Verification items for the finished model (mm, model axes). A direction names the side the tool comes from. Coordinates: 2 decimals unless noted, no trailing zeros. Loops run counter-clockwise (first coordinate to the right, second up) from the corner with the lowest first, then second, coordinate; pieces in that order, holes last. Notation, with made-up numbers: (-17, 58.5) - (22, 58.5) arc R19 cw to (22, 82.5) - close; hole circle Ø4 at (35, 65). An arc over 180 degrees is marked (long way). One line per item, written item: value. Start each with the question number.
(1) Thickness scan on probe 1 along X at (y, z) = (-18.5, 1.5); probe 2 along X at (y, z) = (-6, 2); probe 3 along Y at (x, z) = (47.5, 1.5). Record the ranges inside material, lowest first. Write a range as [from, to].
(2) Section check B-B (x = 33.5). Record the boundary of the cut face in (y, z), plus the area to 3 significant figures.
(3) Section check D-D (z = 1.5). Count the separate pieces of the cut face and the enclosed holes in it, plus the area to 3 significant figures.
(4) Set-up check for faces 5 (the face through (61, -1.707, 1)), 6 (the face through (16.99, 9.74, 1.46)), 7 (the face through (69.238, 16.323, -0.677)), 8 (the face through (24, 9.901, 1)), 9 (the face through (37.1, 12.4, 0)): record each of +Z, -Z, +X, -X, +Y, -Y from which the full face is reachable in a straight line by a thin tool's end or side.
(5) Section check C-C (x = 61.5). Record the boundary of the cut face in (y, z).
(6) Draft check along X on faces 1 (the face through (69.953, 9, 1)), 2 (the face through (25, -1.707, 1)), 3 (the face through (69.24, 9.74, 1.54)), 4 (the face through (61.747, -8.946, 1.351)). Enter one of: +X half, -X half, draft (parallel to the pull), parting line (faces both ways), or undercut.
(7) Gauge pin test, flat ends, axial feed: P1, Ø1, axis at x = 36, y = 18, coming from the +Z side; P2, Ø2, axis at x = 62, z = 1.5, coming from the -Y side; P3, Ø1.5, axis at y = 0, z = 2, coming from the +X side; P4, Ø8, axis at x = 37, y = -7.5, coming from the +Z side. Record the tip position at first contact, or that the pin passes through.
(8) Section check A-A (x = 25). Record the boundary of the cut face in (y, z), plus the area to 3 significant figures.
```python
from build123d import *

# Parameters (mm, degrees)
SKETCH_1_R          = 15
SKETCH_1_R_2        = 1.4
EXTRUDE_1_DEPTH     = 2.74
SKETCH_3_W          = 2.74
SKETCH_3_H          = 6
EXTRUDE_3_DEPTH     = 3.5
SKETCH_11_W         = 2.74
SKETCH_11_H         = 6
EXTRUDE_8_DEPTH     = 3.5
FILLET_17_R         = 2
FILLET_19_R         = 2
CUT_EXTRUDE_1_DEPTH = 1.45
CUT_EXTRUDE_START   = -1.45
CUT_EXTRUDE_2_DEPTH = 1.45


with BuildPart() as part:
    # 草图1 → 凸台-拉伸1 (new body)
    with BuildSketch(Plane.XY):
        with BuildLine():
            Line((25.602982383, 9.901284161), (25.602982383, 3.901284161))
            Line((25.602982383, 3.901284161), (22.865684115, 3.901284161))
            ThreePointArc((22.865684115, 3.901284161), (43.102982383, -22.706902605), (63.340280651, 3.901284161))
            Line((63.340280651, 3.901284161), (60.602982383, 3.901284161))
            Line((60.602982383, 3.901284161), (60.602982383, 9.901284161))
            ThreePointArc((60.602982383, 9.901284161), (43.102982383, 19.293097395), (25.602982383, 9.901284161))
        make_face()
        with Locations((43.102982383, -1.706902605)):
            Circle(SKETCH_1_R, mode=Mode.SUBTRACT)
        with Locations((38.37953481, 15.921243725)):
            Circle(SKETCH_1_R_2, mode=Mode.SUBTRACT)
        with Locations((47.826429956, -19.335048935)):
            Circle(SKETCH_1_R_2, mode=Mode.SUBTRACT)
        with BuildLine():
            Line((26.602982383, -1.706902605), (23.102982383, -1.706902605))
            ThreePointArc((23.102982383, -1.706902605), (28.96084676, -15.849038229), (43.102982383, -21.706902605))
            Line((43.102982383, -21.706902605), (43.102982383, -18.206902605))
            ThreePointArc((43.102982383, -18.206902605), (31.435720494, -13.374164495), (26.602982383, -1.706902605))
        make_face(mode=Mode.SUBTRACT)
        with BuildLine():
            Line((43.102982383, 14.793097395), (43.102982383, 18.12026115))
            ThreePointArc((43.102982383, 18.12026115), (52.478832846, 15.763353566), (59.625618846, 9.252974534))
            Line((59.625618846, 9.252974534), (56.852982383, 7.413815568))
            ThreePointArc((56.852982383, 7.413815568), (50.905486793, 12.831698598), (43.102982383, 14.793097395))
        make_face(mode=Mode.SUBTRACT)
        with BuildLine():
            Line((55.393395475, -12.715796557), (58.000452797, -15.051016486))
            ThreePointArc((58.000452797, -15.051016486), (61.783847035, -8.850101879), (63.102982383, -1.706902605))
            Line((63.102982383, -1.706902605), (59.602982383, -1.706902605))
            ThreePointArc((59.602982383, -1.706902605), (58.514695721, -7.600042006), (55.393395475, -12.715796557))
        make_face(mode=Mode.SUBTRACT)
    extrude(amount=EXTRUDE_1_DEPTH)

    # 草图3 → 凸台-拉伸3 (add)
    with BuildSketch(Plane.ZY.offset(-25.602982383)):
        with Locations((1.37, 6.901284161)):
            Rectangle(SKETCH_3_W, SKETCH_3_H)
    extrude(amount=EXTRUDE_3_DEPTH)

    # 草图11 → 凸台-拉伸8 (add)
    with BuildSketch(Plane(origin=(60.602982383, 0, 0), x_dir=(0, 0, -1), z_dir=(1, 0, 0))):
        with Locations((-1.37, 6.901284161)):
            Rectangle(SKETCH_11_W, SKETCH_11_H)
    extrude(amount=EXTRUDE_8_DEPTH)

    # 圆角17
    # the kernel refuses this fillet: 2 mm, written as the material it adds along each edge
    with BuildSketch(Plane(origin=(63.340280651, 3.901284161, 0), x_dir=(0.228936975336042, -0.9734412469810308, 0), z_dir=(0, 0, 1))) as fillet_17_piece_1:
        with BuildLine():
            CenterArc((1.731032211, 1.998451636), FILLET_17_R, 218.902952144, 48.842355981)
            Line((0.174610628, 0.742445325), (0.143482196, 0.717325199))
            ThreePointArc((0.143482196, 0.717325199), (0.048367664, 0.380380141), (-0.03893765, 0.009157479))
            Line((-0.03893765, 0.009157479), (0.001573666, -0.039969033))
            ThreePointArc((0.001573666, -0.039969033), (0.826174465, -0.023742177), (1.650775263, -0.039969033))
            Line((1.650775263, -0.039969033), (1.652348929, 0))
        make_face()
    extrude(amount=2.74)

    # 圆角19
    # the kernel refuses this fillet: 2 mm, written as the material it adds along each edge
    with BuildSketch(Plane(origin=(22.865684115, 3.901284161, 0), x_dir=(-0.22893697533604487, -0.9734412469810302, 0), z_dir=(0, 0, 1))) as fillet_19_piece_1:
        with BuildLine():
            CenterArc((1.731032211, -1.998451636), FILLET_19_R, 92.254691875, 48.842355981)
            Line((0.174610628, -0.742445325), (0.143482196, -0.717325199))
            ThreePointArc((0.143482196, -0.717325199), (0.048367664, -0.380380141), (-0.03893765, -0.009157479))
            Line((-0.03893765, -0.009157479), (0.001573666, 0.039969033))
            ThreePointArc((0.001573666, 0.039969033), (0.826174465, 0.023742177), (1.650775263, 0.039969033))
            Line((1.650775263, 0.039969033), (1.652348929, 0))
        make_face()
    extrude(amount=2.74)

    # 放样2: read off the stored shape, not the designer's step
    # 放样2: loft between two sections, ruled curve by curve
    loft_2_from = [
        Edge.make_line((64.102982383, 3.901284161, 2.74), (64.102982383, 3.901284161, 0)),
        Edge.make_line((64.102982383, 9.901284161, 2.74), (64.102982383, 3.901284161, 2.74)),
        Edge.make_line((64.102982383, 3.901284161, 0), (64.102982383, 9.901284161, 0)),
        Edge.make_line((64.102982383, 9.901284161, 0), (64.102982383, 9.901284161, 2.74)),
    ]
    loft_2_to = [
        Edge.make_line((69.952982383, 3.901284161, 4.5), (69.952982383, 3.901284161, -1.5)),
        Edge.make_line((69.952982383, 23.901284161, 4.5), (69.952982383, 3.901284161, 4.5)),
        Edge.make_line((69.952982383, 3.901284161, -1.5), (69.952982383, 23.901284161, -1.5)),
        Edge.make_line((69.952982383, 23.901284161, -1.5), (69.952982383, 23.901284161, 4.5)),
    ]
    loft_2 = Solid(Shell([*[Face.make_surface_from_curves(loft_2_from[k], loft_2_to[k]) for k in range(4)], Face(Wire(loft_2_from)), Face(Wire(loft_2_to))]))
    add(loft_2)

    # 草图31 → 切除-拉伸1 (cut)
    with BuildSketch(Plane(origin=(69.952982383, 0, 0), x_dir=(0, 0, -1), z_dir=(1, 0, 0))):
        with BuildLine():
            Line((-1.5, 23.901284161), (-4.125, 23.901284161))
            Line((-4.125, 23.901284161), (-3.4, 11.641284161))
            ThreePointArc((-3.4, 11.641284161), (-1.5, 9.741284161), (0.4, 11.641284161))
            Line((0.4, 11.641284161), (1.125, 23.901284161))
            Line((1.125, 23.901284161), (-1.5, 23.901284161))
        make_face()
    extrude(amount=-CUT_EXTRUDE_1_DEPTH, mode=Mode.SUBTRACT)

    # 放样3: read off the stored shape, not the designer's step
    # 放样3: loft between two sections, ruled curve by curve
    loft_3_from = [
        Edge.make_line((22.102982383, 9.901284161, 0), (22.102982383, 3.901284161, 0)),
        Edge.make_line((22.102982383, 3.901284161, 2.74), (22.102982383, 9.901284161, 2.74)),
        Edge.make_line((22.102982383, 3.901284161, 2.74), (22.102982383, 3.901284161, 0)),
        Edge.make_line((22.102982383, 9.901284161, 2.74), (22.102982383, 9.901284161, 0)),
    ]
    loft_3_to = [
        Edge.make_line((16.252982383, 23.901284161, -1.5), (16.252982383, 3.901284161, -1.5)),
        Edge.make_line((16.252982383, 3.901284161, 4.5), (16.252982383, 23.901284161, 4.5)),
        Edge.make_line((16.252982383, 3.901284161, 4.5), (16.252982383, 3.901284161, -1.5)),
        Edge.make_line((16.252982383, 23.901284161, 4.5), (16.252982383, 23.901284161, -1.5)),
    ]
    loft_3 = Solid(Shell([*[Face.make_surface_from_curves(loft_3_from[k], loft_3_to[k]) for k in range(4)], Face(Wire(loft_3_from)), Face(Wire(loft_3_to))]))
    add(loft_3)

    # 草图32 → 切除-拉伸2 (cut)
    with BuildSketch(Plane.ZY.offset(-16.252982383).offset(CUT_EXTRUDE_START)):
        with BuildLine():
            Line((1.5, 23.901284161), (-1.125, 23.901284161))
            Line((-1.125, 23.901284161), (-0.4, 11.641284161))
            ThreePointArc((-0.4, 11.641284161), (1.5, 9.741284161), (3.4, 11.641284161))
            Line((3.4, 11.641284161), (4.125, 23.901284161))
            Line((4.125, 23.901284161), (1.5, 23.901284161))
        make_face()
    extrude(amount=CUT_EXTRUDE_2_DEPTH, mode=Mode.SUBTRACT)


solid = part.part
```
Responses:
1. probe 1: x = [30.49, 32.24], [43.1, 46.7], [48.95, 55.71]
1. probe 2: x = [22.55, 23.57], [27.17, 28.73], [57.48, 59.03], [62.64, 63.66]
1. probe 3: y = [-22.24, -20.7], [-17.97, -16.05], [12.63, 14.2], [17.63, 18.83]
2. outline: (-20.38, 0) - (-19.25, 0) - (-19.25, 2.74) - (-20.38, 2.74) - close; (-15.12, 0) - (-13.23, 0) - (-13.23, 2.74) - (-15.12, 2.74) - close; (9.82, 0) - (16.97, 0) - (16.97, 2.74) - (9.82, 2.74) - close
2. area: 27.9 mm²
3. separate pieces: 1
3. enclosed holes: 6
3. area: 600 mm²
4. face 5: +Z, -Z
4. face 6: -X, +Y
4. face 7: +X, +Y
4. face 8: +Z, -Z, +Y
4. face 9: -Z, +Y, -Y
5. outline: (-11.83, 0) - (-9.55, 0) - (-9.55, 2.74) - (-11.83, 2.74) - close; (-1.71, 0) - (9.9, 0) - (9.9, 2.74) - (-1.71, 2.74) - close
6. face 1: +X half
6. face 2: undercut
6. face 3: draft
6. face 4: undercut
7. P1: stops at z = 2.74
7. P2: stops at y = -12.69
7. P3: stops at x = 64.08
7. P4: passes through
8. outline: (-12.35, 0) - (-10.21, 0) - (-10.21, 2.74) - (-12.35, 2.74) - close; (-1.71, 0) - (9.9, 0) - (9.9, 2.74) - (-1.71, 2.74) - close
8. area: 37.7 mm²
